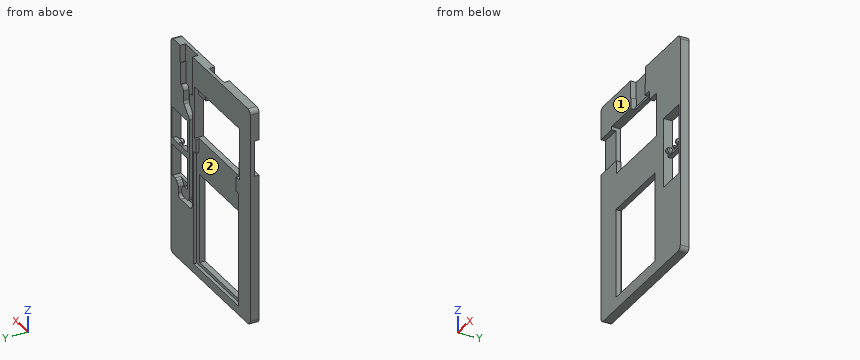
Autodesk Inventor part; units mm, degrees
ref_plane "YZ Plane" through (0, 0, 0) normal (1, 0, 0) x (0, 1, 0)
ref_plane "XZ Plane" through (0, 0, 0) normal (0, 1, 0) x (-1, 0, 0)
ref_plane "XY Plane" through (0, 0, 0) normal (0, 0, 1) x (1, 0, 0)
sketch "Sketch2" plane through (0, 0, 0) normal (0, 1, 0) x (-1, 0, 0)
  line L0 (-33.5, -50) -> (33.5, -50)
  line L1 (33.5, -50) -> (33.5, 50)
  line L2 (33.5, 50) -> (-33.5, 50)
  line L3 (-33.5, 50) -> (-33.5, -50)
  line L4 (-33.5, -50) -> (33.5, 50) construction
  line L5 (33.5, -50) -> (-33.5, 50) construction
  point P0 (0, 0)
  dimension "d0" = 67
  dimension "d1" = 100
extrude "Extrusion1" add sketch "Sketch2" along normal blind 4
sketch "Sketch3" plane through (0, 4, 0) normal (0, 1, 0) x (1, 0, 0)
  line L0 (33.5, 50) -> (-33.5, 50)
  line L1 (-23.5, -6.5) -> (14.5, -6.5)
  line L2 (14.5, -6.5) -> (14.5, 46)
  line L3 (14.5, 46) -> (-23.5, 46)
  line L4 (-23.5, 46) -> (-23.5, -6.5)
  line L5 (-23.5, -6.5) -> (14.5, 46) construction
  line L6 (14.5, -6.5) -> (-23.5, 46) construction
  line L7 (-33.5, 50) -> (-33.5, -50)
  point P0 (0, 0)
  point P1 (-4.5, 19.75)
  dimension "d4" = 38
  dimension "d5" = 52.5
  dimension "d6" = 4
  dimension "d111" = 10
extrude "Extrusion2" cut sketch "Sketch3" against normal blind 1.5
sketch "Sketch4" plane through (0, 2.5, 0) normal (0, 1, 0) x (1, 0, 0)
  line L0 (14.5, -6.5) -> (-23.5, -6.5)
  line L1 (14.5, 46) -> (14.5, -6.5)
  line L2 (-23.5, 46) -> (14.5, 46)
  line L3 (-23.5, -6.5) -> (-23.5, 46)
  line L4 (-21, 44.5) -> (12, 44.5)
  line L5 (12, 44.5) -> (12, 3.5)
  line L6 (12, 3.5) -> (-21, 3.5)
  line L7 (-21, 3.5) -> (-21, 44.5)
  line L8 (-21, 44.5) -> (12, 3.5) construction
  line L9 (12, 44.5) -> (-21, 3.5) construction
  point P0 (0, 0)
  point P1 (-4.5, 24)
  dimension "d9" = 10
  dimension "d10" = 1.5
  dimension "d11" = 2.5
  dimension "d12" = 2.5
extrude "Extrusion3" cut sketch "Sketch4" against normal blind 2.5 contours L4 L5 L6 L7
sketch "Sketch12" plane through (0, 4, 0) normal (0, 1, 0) x (1, 0, 0)
  line L0 (-24.5, -37) -> (13.5, -37)
  line L1 (13.5, -37) -> (13.5, -13)
  line L2 (13.5, -13) -> (-24.5, -13)
  line L3 (-24.5, -13) -> (-24.5, -37)
  line L4 (-24.5, -37) -> (13.5, -13) construction
  line L5 (13.5, -37) -> (-24.5, -13) construction
  line L6 (-23.5, -6.5) -> (-23.5, 46)
  line L7 (14.5, -6.5) -> (-23.5, -6.5)
  point P0 (0, 0)
  point P1 (-5.5, -25)
  point P2 (-5.5, -25)
  dimension "d58" = 38
  dimension "d59" = 24
  dimension "d112" = 1
  dimension "d154" = 6.5
extrude "Extrusion10" cut sketch "Sketch12" against normal blind 4
sketch "Sketch18" plane through (13.5, 4, 13) normal (-1, 0, 0) x (0, 0, 1)
  line L0 (0, 0) -> (24, 0)
  line L1 (24, -4) -> (20, -4)
  line L2 (20, -4) -> (20, -1.8)
  line L3 (20, -1.8) -> (24, -1.8)
  line L4 (24, -1.8) -> (24, -4)
  point P0 (-13, -4)
  dimension "d88" = 4
  dimension "d89" = 1.8
extrude "Extrusion17" add sketch "Sketch18" along normal blind 6
sketch "Sketch20" plane through (-24.5, 4, 37) normal (1, 0, 0) x (0, 0, -1)
  line L0 (0, 0) -> (24, 0)
  line L1 (24, -4) -> (18, -4)
  line L2 (18, -4) -> (18, -1.8)
  line L3 (18, -1.8) -> (24, -1.8)
  line L4 (24, -1.8) -> (24, -4)
  point P0 (37, -4)
  dimension "d96" = 6
  dimension "d97" = 1.8
extrude "Extrusion19" add sketch "Sketch20" along normal blind 4
sketch "Sketch22" plane through (0, 0, 0) normal (0, -1, 0) x (1, 0, 0)
  line L0 (33.5, 50) -> (33.5, -50)
  line L1 (32.5, -14) -> (19.5, -14)
  line L2 (19.5, -14) -> (19.5, 18)
  line L3 (19.5, 18) -> (32.5, 18)
  line L4 (32.5, 18) -> (32.5, -14)
  line L5 (33.5, -50) -> (-33.5, -50)
  point P0 (0, 0)
  dimension "d102" = 1
  dimension "d103" = 13
  dimension "d110" = 32
  dimension "d155" = 36
extrude "Extrusion21" cut sketch "Sketch22" against normal up to next
sketch "Sketch23" plane through (0, 4, 0) normal (0, 1, 0) x (1, 0, 0)
  line L0 (-24.5, -13) -> (13.5, -13)
  line L1 (14.5, 46) -> (14.5, -6.5)
  line L2 (14.5, -6.5) -> (-23.5, -6.5)
  line L3 (-23.5, -6.5) -> (-23.5, 46)
  line L4 (-21.5, -6.5) -> (-21.5, -13)
  line L5 (12.5, -6.5) -> (12.5, -13)
  point P0 (0, 0)
  dimension "d114" = 2
  dimension "d115" = 2
extrude "Extrusion22" cut sketch "Sketch23" against normal up to surface (1.5 mm away)
sketch "Sketch24" plane through (32.5, 0, -14) normal (-1, 0, 0) x (0, 0, 1)
  line L0 (0, 0) -> (0, 4)
  line L1 (14.5, 2) -> (17.5, 2)
  line L2 (17.5, 2) -> (17.5, 4)
  line L3 (17.5, 4) -> (14.5, 4)
  line L4 (14.5, 4) -> (14.5, 2)
  line L5 (14.5, 2) -> (17.5, 4) construction
  line L6 (17.5, 2) -> (14.5, 4) construction
  line L7 (0, 4) -> (32, 4)
  point P0 (16, 3)
  dimension "d118" = 3
  dimension "d119" = 2
  dimension "d120" = 16
extrude "Extrusion23" add sketch "Sketch24" along normal up to next
sketch "Sketch25" plane through (32.5, 2, 0.5) normal (0, -1, 0) x (1, 0, 0)
  line L0 (-8, 1) -> (-5, 1)
  line L1 (-5, 1) -> (-5, 3)
  line L2 (-5, 3) -> (-8, 3)
  line L3 (-8, 3) -> (-8, 1)
  line L4 (-8, 1) -> (-5, 3) construction
  line L5 (-5, 1) -> (-8, 3) construction
  line L6 (0, 3) -> (-13, 3)
  point P0 (32.5, 26.5)
  point P1 (-6.5, 2)
  point P2 (-6.5, 2)
  point P3 (-6.5, 0)
  point P4 (-6.5, 2)
  point P5 (-6.5, 3)
  dimension "d123" = 3
  dimension "d124" = 2
extrude "Extrusion24" cut sketch "Sketch25" against normal blind 0.5
fillet "Fillet6" radius 1 1 edges at (26, 2.5, 3.5)
sketch "Sketch26" plane through (32.5, 2, 0.5) normal (0, -1, 0) x (1, 0, 0)
  line L0 (0, 3) -> (0, 0)
  circle A0 centre (-10.625, 1.5) radius 1.25
  circle A1 centre (-2.375, 1.5) radius 1.25
  line L1 (0, 3) -> (-13, 3)
  line L2 (-13, -14.5) -> (-13, 17.5)
  point P0 (32.5, 26.5)
  point P1 (-6.5, 1.5)
  point P2 (0, 1.5)
  point P3 (-6.5, 0)
  point P4 (-6.5, 3)
  point P5 (-13, 1.5)
  dimension "d128" = 2.5
  dimension "d129" = 2.5
  dimension "d130" = 4.125
  dimension "d131" = 8.25
extrude "Extrusion25" add sketch "Sketch26" along normal blind 2
chamfer "Chamfer3" distance 0.5 angle 45 2 edges at (28.875, 0, 2) (20.625, 0, 2)
sketch "Sketch27" plane through (0, 4, 0) normal (0, 1, 0) x (1, 0, 0)
  line L0 (-33.5, -50) -> (33.5, -50)
  line L1 (32.5, -18) -> (19.5, -18)
  line L2 (19.5, 14) -> (32.5, 14)
  line L3 (15.25, -50) -> (25.75, -50)
  line L4 (25.75, -50) -> (25.75, -32)
  line L5 (25.75, -32) -> (15.25, -32)
  line L6 (15.25, -32) -> (15.25, -50)
  line L7 (15.25, -50) -> (25.75, -32) construction
  line L8 (25.75, -50) -> (15.25, -32) construction
  line L9 (19.5, -18) -> (19.5, 14)
  line L10 (15.25, -42) -> (15.5, -42)
  line L11 (15.5, -42) -> (15.5, -32)
  line L12 (25.75, -42) -> (25.5, -42)
  line L13 (25.5, -42) -> (25.5, -32)
  point P0 (0, 0)
  point P1 (26, 14)
  point P2 (20.5, -41)
  point P3 (20.5, -41)
  point P4 (26, -18)
  dimension "d138" = 10.5
  dimension "d139" = 18
  dimension "d148" = 0.25
  dimension "d149" = 0.25
  dimension "d150" = 8
  dimension "d168" = 13
extrude "Extrusion26" cut sketch "Sketch27" against normal blind 2.5 contours L6 L10 L11 L5 L13 L12 L4 L0
sketch "Sketch29" plane through (0, 0, 0) normal (0, -1, 0) x (1, 0, 0)
  line L0 (-24.5, 19) -> (-24.5, 37)
  line L1 (-24.5, 37) -> (7.5, 37)
  line L2 (-33.5, -50) -> (-33.5, 50)
  line L3 (-33.5, 50) -> (33.5, 50)
  line L4 (-24.5, 19) -> (-33.5, 19)
  line L5 (-24.5, 35.5) -> (-33.5, 35.5)
  point P0 (0, 0)
  dimension "d151" = 1.5
extrude "Extrusion28" cut sketch "Sketch29" against normal blind 2
sketch "Sketch30" plane through (0, 0, 0) normal (0, -1, 0) x (1, 0, 0)
  line L0 (-33.5, 50) -> (33.5, 50)
  line L1 (-8.5, 42) -> (4, 42)
  line L2 (4, 42) -> (4, 50)
  line L3 (4, 50) -> (-8.5, 50)
  line L4 (-8.5, 50) -> (-8.5, 42)
  line L5 (-8.5, 42) -> (4, 50) construction
  line L6 (4, 42) -> (-8.5, 50) construction
  line L7 (3.75, 37) -> (-8.25, 37)
  line L8 (-8.25, 37) -> (-8.25, 42)
  line L9 (-8.25, 42) -> (3.75, 42)
  line L10 (3.75, 42) -> (3.75, 37)
  line L11 (3.75, 37) -> (-8.25, 42) construction
  line L12 (-8.25, 37) -> (3.75, 42) construction
  line L13 (-24.5, 37) -> (7.5, 37)
  point P0 (0, 0)
  point P1 (-2.25, 46)
  point P2 (-2.25, 39.5)
  point P3 (-2.25, 39.5)
  point P4 (-2.25, 46)
  dimension "d156" = 12.5
  dimension "d157" = 8
  dimension "d158" = 16
  dimension "d162" = 12
extrude "Extrusion29" cut sketch "Sketch30" against normal blind 2.5
sketch "Sketch32" plane through (0, 2.5, 0) normal (0, -1, 0) x (1, 0, 0)
  line L0 (-8.25, 37) -> (-8.25, 42)
  line L1 (3.75, 37) -> (-8.25, 37)
  line L2 (3.75, 42) -> (3.75, 37)
  line L3 (-8.25, 42) -> (-8.5, 42)
  line L4 (-8.25, 38) -> (3.75, 38)
  point P0 (0, 0)
  dimension "d183" = 1
extrude "Extrusion31" add sketch "Sketch32" along normal blind 0.5
sketch "Sketch33" plane through (0, 4, 0) normal (0, 1, 0) x (1, 0, 0)
  line L0 (27.25, 14) -> (27.25, 21.5)
  line L1 (27.25, 21.5) -> (15.5, 21.5)
  line L2 (15.5, 21.5) -> (15.5, -24.5)
  line L3 (24.75, 14) -> (24.75, 19)
  line L4 (24.75, 19) -> (18, 19)
  line L5 (18, 19) -> (18, -19.9289)
  line L6 (18, -19.9289) -> (23, -24.9289)
  line L7 (23, -24.9289) -> (23, -32)
  line L8 (15.5, -24.5) -> (18, -27)
  line L9 (18, -27) -> (18, -32)
  line L10 (19.5, 14) -> (32.5, 14)
  line L11 (18, -32) -> (23, -32)
  line L12 (24.75, 14) -> (27.25, 14)
  line L13 (15.5, -32) -> (25.5, -32)
  line L14 (13.5, -13) -> (13.5, -37)
  point P0 (0, 0)
  point P1 (26, 14)
  point P2 (20.5, -32)
  point P3 (20.5, -32)
  point P4 (26, 14)
  point P5 (20.5, -32)
  dimension "d198" = 2.5
  dimension "d199" = 2.5
  dimension "d200" = 2.5
  dimension "d201" = 5
  dimension "d202" = 5
  dimension "d203" = 135
  dimension "d204" = 135
  dimension "d205" = 2.5
  dimension "d206" = 1.25
  dimension "d207" = 2
  dimension "d208" = 5
  dimension "d209" = 5
extrude "Extrusion32" cut sketch "Sketch33" against normal up to surface (2.5 mm away)
chamfer "Chamfer6" distance 2 angle 45 2 edges at (24.75, 2.75, -14) (27.25, 2.75, -14)
fillet "Fillet9" radius 2 13 edges at (22.75, 2.75, -14) (27.25, 2.75, -16) (29.25, 2.75, -14) (27.25, 2.75, -21.5) (15.5, 2.75, -21.5) (18, 2.75, 19.9289) (23, 2.75, 24.9289) (23, 2.75, 32) (18, 2.75, 32) (18, 2.75, 27) (15.5, 2.75, 24.5) (24.75, 2.75, -16) (24.75, 2.75, -19)
fillet "Fillet9" radius 2 1 edges at (18, 2.75, -19)
fillet "Fillet10" radius 2 4 edges at (33.5, 2, 50) (-33.5, 2, 50) (33.5, 2, -50) (-33.5, 2, -50)
properties part number "DisplayBottom2"
Design review of the part built by this model. Coordinates are the model's own, in mm. Face numbers are marked on the shaded views. Give positions to 0.01 mm unless a question says otherwise; leave off trailing zeros. Write each loop counter-clockwise with the first axis right and the second up, starting at its lowest first coordinate (ties: lowest second). Pieces come first, ordered by that corner, then holes. Notation, with made-up numbers: (30.5, -27.75) -> (70.5, -27.75) arc R30 cw to (70.5, -2.75) -> close; hole circle Ø9 at (36, -18). An arc over 180 degrees is marked (long way). Answer in a Markdown table with one row per item.
(1) Clearance check with flat-ended pins moving along their axes: pin 1 (1.2 mm diameter, centred on x = -5.5, y = 1, fed in from +Z); pin 2 (3 mm diameter, centred on x = -7.5, z = 9, fed in from +Y); pin 3 (0.8 mm diameter, centred on x = -2, z = 37.5, fed in from -Y). State where each tip first meets the part, or that it passes through.
Results:
| item | result |
|---|---|
| pin 1 | z = 13 |
| pin 2 | y = 2.5 |
| pin 3 | y = 2 |
(2) Consider section D-D (z = 21.5). State the section outline as (x, y) points, then the cut area to 3 significant figures.
Results:
| item | result |
|---|---|
| outline | (-33.5, 2) -> (-24.5, 2) -> (-24.5, 4) -> (-33.5, 4) -> close; (13.5, 0) -> (33.5, 0) -> (33.5, 4) -> (19.57, 4) -> (19.57, 1.5) -> (15.5, 1.5) -> (15.5, 4) -> (13.5, 4) -> close |
| area | 87.8 mm2 |
(3) Consider section A-A (z = -26.5). State the section outline as (x, y) points.
Results:
| item | result |
|---|---|
| outline | (-33.5, 0) -> (-21, 0) -> (-21, 2.5) -> (-23.5, 2.5) -> (-23.5, 4) -> (-33.5, 4) -> close; (12, 0) -> (33.5, 0) -> (33.5, 4) -> (14.5, 4) -> (14.5, 2.5) -> (12, 2.5) -> close |
(4) Mouldability with a two-part tool opening along X and no side actions: class the marked faces 1 and 2 as +X half, -X half, draft (parallel to the pull), parting line (faces both ways), or undercut.
Results:
| item | result |
|---|---|
| face 1 | draft |
| face 2 | undercut |
(5) To check wall thickness, follow probe 1 along Z at (x, y) = (6, 2.25); probe 2 along X at (y, z) = (0.7, -9); probe 3 along Z at (x, y) = (30, 3.45). State the ranges of each line that lie inside material, in increasing order.
Results:
| item | result |
|---|---|
| probe 1 | -50 to -44.5, -3.5 to 13, 37 to 50 |
| probe 2 | -33.5 to -21, 12 to 19.5, 32.5 to 33.5 |
| probe 3 | -50 to -14, 0.5 to 3.5, 18 to 50 |
(6) Consider section C-C (x = -0.5). State the section outline as (y, z) points, then the cut area to 3 significant figures.
Results:
| item | result |
|---|---|
| outline | (0, -50) -> (4, -50) -> (4, -46) -> (2.5, -46) -> (2.5, -44.5) -> (0, -44.5) -> close; (0, -3.5) -> (2.5, -3.5) -> (2.5, 13) -> (0, 13) -> close; (2, 37) -> (4, 37) -> (4, 50) -> (2.5, 50) -> (2.5, 38) -> (2, 38) -> close |
| area | 81.0 mm2 |
(7) Consider section B-B (x = -15). State the section outline as (y, z) points, then the cut area to 3 significant figures.
Results:
| item | result |
|---|---|
| outline | (0, -50) -> (4, -50) -> (4, -46) -> (2.5, -46) -> (2.5, -44.5) -> (0, -44.5) -> close; (0, -3.5) -> (2.5, -3.5) -> (2.5, 13) -> (0, 13) -> close; (0, 37) -> (4, 37) -> (4, 50) -> (0, 50) -> close |
| area | 113 mm2 |
